```python
from build123d import *

# Parameters (mm, degrees)
SKETCH_R      = 9
SKETCH_R_2    = 0.6
PAD_DEPTH     = 2
SKETCH001_R   = 10.2
SKETCH001_R_2 = 9
PAD001_DEPTH  = 5


with BuildPart() as part:
    # Sketch → Pad (new body)
    with BuildSketch(Plane.XY):
        Polygon((-0.50397, 14.713397), (-12.984903, 7.508821), (-12.99, -7.5), (0, -14.99967), (12.99, -7.5), (12.99, 7.5), (12.74, 7.066987), align=None)
        Circle(SKETCH_R, mode=Mode.SUBTRACT)
        with Locations((5.975274, 9.914229)):
            Circle(SKETCH_R_2, mode=Mode.SUBTRACT)
    extrude(amount=PAD_DEPTH)

    # Sketch001 (on Face10 of Pad) → Pad001 (join)
    with BuildSketch(Plane(origin=(0, 0, 0), x_dir=(1, 0, 0), z_dir=(0, 0, -1))):
        Circle(SKETCH001_R)
        Circle(SKETCH001_R_2, mode=Mode.SUBTRACT)
    extrude(amount=PAD001_DEPTH)


solid = part.part
```
Work out the finished part from the listing and answer in its coordinate system (mm). A direction names the side the tool comes from. Coordinates: 2 decimals unless noted, no trailing zeros. Loops run counter-clockwise (first coordinate to the right, second up) from the corner with the lowest first, then second, coordinate; pieces in that order, holes last. Notation, with made-up numbers: M 10.5,-19.75 L 21.5,-19.75 A10 cw 21.5,-0.75 Z; hole C 70,29.5 d3. An arc over 180 degrees is marked long. Use CSV: the item, a comma, the result in double quotes. Start each with the question number.
(1) Consider line 1 (X direction, y = 0, z = -1.75); line 2 (Y direction, x = 5.5, z = 1.5); line 3 (Y direction, x = 6, z = 0.25). Determine where each line is inside the solid, lowest interval first.
(2) For faces 1 (the face through (12.99, 0, 1)), 2 (the face through (-3, -10, 0)), determine the directions among +Z, -Z, +X, -X, +Y, -Y from which every point of the face is accessible in a straight line to the end or side of a thin tool.
(3) Find section B-B, the plane z = 0.75. Give the vertices of the cut face in (x, y).
(4) Given pin 1 Ø6 at (x, y) = (-7.5, -4) entering from +Z; pin 2 Ø3 at (x, z) = (-5.5, -3.5) entering from -Y, each flat-ended and moving along its own axis, determine where each tip first touches the part or whether it passes through.
(5) Find section D-D, the plane z = -2.25. Give the vertices of the cut face in (x, y), then the cut area to 3 significant figures.
(6) Find section C-C, the plane x = 7. Give the vertices of the cut face in (y, z), then the cut area to 3 significant figures.
(7) For a pull along X with two mould halves and no side action, classify faces 3 (the face through (-1.172, -8.923, -1.451)), 4 (the face through (-6.586, -11.197, 0.986)), 5 (the face through (4.707, 9.049, -2.465)), 6 (the face through (0, -10, 2)) as +X half, -X half, draft (parallel to the pull), parting line (faces both ways), or undercut.
(8) Find section A-A, the plane y = 0. Give the vertices of the cut face in (x, z), then the cut area to 3 significant figures.
Recorded:
1,line 1,"x = -10.2 to -9, 9 to 10.2"
1,line 2,"y = -11.82 to -7.12, 7.12 to 9.55, 10.28 to 11.25"
1,line 3,"y = -11.54 to -6.71, 6.71 to 9.31, 10.51 to 10.96"
2,face 1,"+Z, -Z, +X, +Y, -Y"
2,face 2,"-Z"
3,outline,"M -12.99,-7.5 L 0,-15 L 12.99,-7.5 L 12.99,7.5 L 12.74,7.07 L -0.5,14.71 L -12.98,7.51 Z; hole C 0,0 d18; hole C 5.98,9.91 d1.2"
4,pin 1,"stops at z = 2"
4,pin 2,"stops at y = -9.38"
5,outline,"C 0,0 d20.4; hole C 0,0 d18"
5,area,"72.4 mm^2"
6,outline,"M -10.96,0 L -7.42,0 L -7.42,-5 L -5.66,-5 L -5.66,2 L -10.96,2 Z; M 5.66,-5 L 7.42,-5 L 7.42,0 L 10.38,0 L 10.38,2 L 5.66,2 Z"
6,area,"37.7 mm^2"
7,face 3,"undercut"
7,face 4,"-X half"
7,face 5,"parting line"
7,face 6,"draft"
8,outline,"M -12.99,0 L -10.2,0 L -10.2,-5 L -9,-5 L -9,2 L -12.99,2 Z; M 9,-5 L 10.2,-5 L 10.2,0 L 12.99,0 L 12.99,2 L 9,2 Z"
8,area,"28.0 mm^2"
